The listing builds one solid part. Answer for the finished solid, in the listing's coordinates (mm). A direction names the side the tool comes from. Give positions to 0.01 mm unless a question says otherwise; leave off trailing zeros. Write each loop counter-clockwise with the first axis right and the second up, starting at its lowest first coordinate (ties: lowest second). Pieces come first, ordered by that corner, then holes. Notation, with made-up numbers: (-38.5, 42.25) - (1.5, 42.25) arc R34 ccw to (1.5, 78.25) - close; hole circle Ø5 at (88, 14.25). An arc over 180 degrees is marked (long way). One line per question, with ' | ' between items. Start each with the question number.
1. Given P1, Ø15, axis at x = 0, z = 354, coming from the +Y side; P2, Ø18, axis at y = -95, z = 358, coming from the -X side; P3, Ø4, axis at x = 244.5, z = 102.5, coming from the +Y side, each flat-ended and moving along its own axis, determine where each tip first touches the part or whether it passes through.
2. A cutting plane is placed at B-B (y = -100). Determine the outline of the cut face in (x, z), then the cut area to 3 significant figures.
3. The mould has two halves that part along Z. Classify faces 1 (the face through (1, -95, 400)), 2 (the face through (5.42, -124.406, 198.6)), 3 (the face through (0, -55, 350)), 4 (the face through (196, 4, 0)): +Z half, -Z half, draft (parallel to the pull), parting line (faces both ways), or undercut.
4. For faces 5 (the face through (-50, -95, 351)), 6 (the face through (247, 300, 49)), 7 (the face through (1, -125, 349)), 8 (the face through (12, -65, 338)), 9 (the face through (50, -95, 349)), determine the directions among +Z, -Z, +X, -X, +Y, -Y from which every point of the face is accessible in a straight line to the end or side of a thin tool.
5. A cutting plane is placed at C-C (x = 370). Determine the outline of the cut face in (y, z).
6. A cutting plane is placed at A-A (z = 350). Determine the outline of the cut face in (x, y).
7. A cutting plane is placed at D-D (y = -26). Determine the outline of the cut face in (x, z).
8. Find the intervals of material crossed by L1, parallel to Z at x = 435, y = 175.5; L2, parallel to Y at x = -1, z = 305.5; L3, parallel to X at y = -94, z = 328, in increasing order. Write a range as from..to.
Autodesk Fusion 360 part; units mm, degrees
sketch "Sketch1" plane through (0, 0, 0) normal (0, 0, 1) x (1, 0, 0)
  line L0 (0, 300) -> (500, 300)
  line L1 (0, -300) -> (500, -300)
  line L2 (0, 300) -> (-100, 0)
  line L3 (-100, 0) -> (0, -300)
  line L4 (500, 300) -> (500, -300)
  dimension "d1" = 500
extrude "Extrude1" add sketch "Sketch1" along normal blind 100
sketch "Sketch2" plane through (0, 0, 100) normal (0, 0, 1) x (-1, 0, 0)
  line L0 (0, -300) -> (100, 0)
  line L1 (100, 0) -> (0, 300)
  line L2 (0, 300) -> (-500, 300)
  line L3 (-500, 300) -> (-500, -300)
  line L4 (-500, -300) -> (0, -300)
  circle A0 centre (0, 100) radius 25
  circle A1 centre (0, -100) radius 25
  dimension "d7" = 50
  dimension "d8" = 50
extrude "Extrude2" add sketch "Sketch2" along normal blind 265 contours A0
ref_plane "WorkPlane1" through (0, -125, 274.5445) normal (0, -1, 0) x (-1, 0, 0)
sketch "Sketch3" plane through (0, -125, 0) normal (0, -1, 0) x (-1, 0, 0)
  line L0 (50, -300) -> (-50, -300)
  line L1 (-50, -300) -> (-50, -400)
  line L2 (-50, -400) -> (50, -400)
  line L3 (50, -400) -> (50, -300)
extrude "Extrude3" add sketch "Sketch3" against normal blind 60
sketch "Sketch4" plane through (0, -65, 0) normal (0, 1, 0) x (-1, 0, 0)
  line L0 (50, 300) -> (50, 400)
  line L1 (50, 400) -> (-50, 400)
  line L2 (-50, 400) -> (-50, 300)
  line L3 (-50, 300) -> (50, 300)
  circle A0 centre (0, 350) radius 15
  dimension "d14" = 30
extrude "Extrude4" add sketch "Sketch4" along normal blind 10 contours A0
Determined:
1) P1: y = -55 | P2: x = -50 | P3: through
2) outline: (-66.67, 0) - (500, 0) - (500, 100) - (25, 100) - (25, 300) - (50, 300) - (50, 400) - (-50, 400) - (-50, 300) - (-25, 300) - (-25, 100) - (-66.67, 100) - close | area: 76,700 mm2
3) face 1: +Z half | face 2: undercut | face 3: draft | face 4: -Z half
4) face 5: +Z, -X, +Y, -Y | face 6: +Z, -Z, +X, -X, +Y | face 7: +Z, +X, -X, -Y | face 8: +Y | face 9: +Z, +X, +Y, -Y
5) outline: (-300, 0) - (300, 0) - (300, 100) - (-300, 100) - close
6) outline: (-50, -125) - (50, -125) - (50, -65) - (15, -65) - (15, -55) - (-15, -55) - (-15, -65) - (-50, -65) - close
7) outline: (-91.33, 0) - (500, 0) - (500, 100) - (-91.33, 100) - close
8) L1: 0..100 | L2: -125..-65 | L3: -50..50
